from build123d import *

# Parameters (mm, degrees)
BOSS_EXTRU_1_DEPTH           = 10
BOSS_EXTRU_2_DEPTH           = 10
ESQUISSE4_R                  = 1.6
ENL_V_MAT_EXTRU_1_DEPTH      = 15
ESQUISSE5_R                  = 2.05
ENL_V_MAT_EXTRU_2_DEPTH      = 15
CONG_1_R                     = 2.5
ESQUISSE6_W                  = 10
ESQUISSE6_H                  = 2
BOSS_EXTRU_3_DEPTH           = 10
CHANFREIN1_SIZE              = 10
CONG_1_OF_SYM_TRIE1_R        = 2.5
CHANFREIN1_OF_SYM_TRIE1_SIZE = 10


with BuildPart() as part:
    # Esquisse2 → Boss.-Extru.1 (new body)
    with BuildSketch(Plane.XY):
        Polygon((125, 17.5), (125, 7.5), (20, 7.5), (20, 17.5), (15, 17.5), (15, 7.5), (0, 7.5), (0, -7.5), (125, -7.5), (125, -17.5), (130, -17.5), (130, 17.5), align=None)
    boss_extru_1 = extrude(amount=BOSS_EXTRU_1_DEPTH)

    # Esquisse3 → Boss.-Extru.2 (add)
    with BuildSketch(Plane.XY.offset(10)):
        Polygon((125, 7.5), (125, -7.5), (125, -17.5), (130, -17.5), (130, 17.5), (125, 17.5), align=None)
    boss_extru_2 = extrude(amount=BOSS_EXTRU_2_DEPTH)

    # Esquisse4 → Enlèv. mat.-Extru.1 (cut)
    with BuildSketch(Plane.ZY.offset(-15)):
        with Locations((5, 12.5)):
            Circle(ESQUISSE4_R)
    enl_v_mat_extru_1 = extrude(amount=-ENL_V_MAT_EXTRU_1_DEPTH, mode=Mode.SUBTRACT)

    # Esquisse5 → Enlèv. mat.-Extru.2 (cut)
    with BuildSketch(Plane.ZY.offset(-125)):
        with Locations(Location((10, 12.5, 0), (0, 0, 270))):
            Circle(ESQUISSE5_R)
        with Locations(Location((10, -12.5, 0), (0, 0, 180))):
            Circle(ESQUISSE5_R)
    enl_v_mat_extru_2 = extrude(amount=-ENL_V_MAT_EXTRU_2_DEPTH, mode=Mode.SUBTRACT)

    # Congé1
    cong_1_edges = [part.edges().sort_by_distance(p)[0] for p in [
        (127.5, 17.5, 0),
        (17.5, 17.5, 10),
        (127.5, -17.5, 0),
        (62.5, -7.5, 0),
        (7.5, 7.5, 0),
        (17.5, 17.5, 0),
        (72.5, 7.5, 0),
        (7.5, 7.5, 10),
        (62.5, -7.5, 10),
        (127.5, -17.5, 20),
        (127.5, 17.5, 20),
        (72.5, 7.5, 10),
    ]]
    fillet(cong_1_edges, radius=CONG_1_R)

    # Esquisse6 → Boss.-Extru.3 (add)
    with BuildSketch(Plane.ZY.offset(-125)):
        with Locations((15, 1)):
            Rectangle(ESQUISSE6_W, ESQUISSE6_H)
        with Locations((15, -1)):
            Rectangle(ESQUISSE6_W, ESQUISSE6_H)
    boss_extru_3 = extrude(amount=BOSS_EXTRU_3_DEPTH)

    # Chanfrein1
    chanfrein1_edges = [part.edges().sort_by_distance(p)[0] for p in [
        (115, 0, 20),
    ]]
    chamfer(chanfrein1_edges, length=CHANFREIN1_SIZE - 0.0001)  # a hair under: the kernel refuses the full size

    # Symétrie1: Boss.-Extru.1, Boss.-Extru.2, Enlèv. mat.-Extru.1, Enlèv. mat.-Extru.2, Boss.-Extru.3 across plane
    add(boss_extru_1.mirror(Plane(origin=(0, 0, 0), x_dir=(0, 0, 1), z_dir=(1, 0, 0))))
    add(boss_extru_2.mirror(Plane(origin=(0, 0, 0), x_dir=(0, 0, 1), z_dir=(1, 0, 0))))
    add(enl_v_mat_extru_1.mirror(Plane(origin=(0, 0, 0), x_dir=(0, 0, 1), z_dir=(1, 0, 0))), mode=Mode.SUBTRACT)
    add(enl_v_mat_extru_2.mirror(Plane(origin=(0, 0, 0), x_dir=(0, 0, 1), z_dir=(1, 0, 0))), mode=Mode.SUBTRACT)
    add(boss_extru_3.mirror(Plane(origin=(0, 0, 0), x_dir=(0, 0, 1), z_dir=(1, 0, 0))))

    # Congé1 of Symétrie1
    cong_1_of_sym_trie1_edges = [part.edges().sort_by_distance(p)[0] for p in [
        (-127.5, 17.5, 0),
        (-17.5, 17.5, 10),
        (-127.5, -17.5, 0),
        (-62.5, -7.5, 0),
        (-7.5, 7.5, 0),
        (-17.5, 17.5, 0),
        (-72.5, 7.5, 0),
        (-7.5, 7.5, 10),
        (-62.5, -7.5, 10),
        (-127.5, -17.5, 20),
        (-127.5, 17.5, 20),
        (-72.5, 7.5, 10),
    ]]
    fillet(cong_1_of_sym_trie1_edges, radius=CONG_1_OF_SYM_TRIE1_R)

    # Chanfrein1 of Symétrie1
    chanfrein1_of_sym_trie1_edges = [part.edges().sort_by_distance(p)[0] for p in [
        (-115, 0, 20),
    ]]
    chamfer(chanfrein1_of_sym_trie1_edges, length=CHANFREIN1_OF_SYM_TRIE1_SIZE - 0.0001)  # a hair under: the kernel refuses the full size


solid = part.part
The model under review builds one solid part; all positions refer to its coordinate system, in mm. A direction names the side the tool comes from. Give positions to 0.01 mm unless a question says otherwise; leave off trailing zeros. Order: outer loops, then holes, each group sorted by start corner. A loop starts at its lowest first (then second) coordinate and runs counter-clockwise, first axis right, second up. Notation, with made-up numbers: M -22,83 L -15,83 A17 cw -15,106 Z; hole C 63.5,-19 d1. An arc over 180 degrees is marked long. Answer in a Markdown table with one row per item. Add a question column.
1. For pin 1 Ø10 at (x, z) = (23.5, 10.5) entering from -Y; pin 2 Ø8 at (x, z) = (-121.5, 16) entering from +Y; pin 3 Ø12 at (x, z) = (62, 14) entering from +Y; pin 4 Ø5 at (x, z) = (-79, 6) entering from +Y, all flat-tipped, find the tip position at first contact; note any pin that passes through.
2. Machinability: for faces 1 (the flat face through (-121, 2, 14)), 2 (the flat face through (2, -7.5, 5)), 3 (the flat face through (73, 7.5, 5)), 4 (the cylindrical face through (-127.465, 14.127, 8.753)), which of the approach directions +Z, -Z, +X, -X, +Y, -Y give a long, thin tool a straight path to every point of the face, cutting with its end or side? Answer none if there is none.
3. Mouldability with a two-part tool opening along Y and no side actions: class faces 5 (the flat face through (-15, 11, 4)), 6 (the flat face through (121, -2, 14)), 7 (the cylindrical face through (127.465, 14.127, 8.753)) as released by +Y, released by -Y, zero draft, split by the parting line, or undercut.
4. Add section A-A on x = -54.5. State the section outline as (y, z) points, plus the area to 3 significant figures.
5. To check wall thickness, follow line 1 along Y through (x, z) = (-127.8, 10); line 2 along X through (y, z) = (15, 5.25); line 3 along X through (y, z) = (6, 12.25). State the ranges of each line that lie inside material, in increasing order.
The answers:
| question | item | result |
|---|---|---|
| 1 | pin 1 | y = -7.5 |
| 1 | pin 2 | y = 17.5 |
| 1 | pin 3 | y = 7.45 |
| 1 | pin 4 | y = 7.5 |
| 2 | face 1 | +Z, +Y |
| 2 | face 2 | +Z, -Z, -Y |
| 2 | face 3 | +Z, -Z, +Y |
| 2 | face 4 | -X |
| 3 | face 5 | zero draft |
| 3 | face 6 | released by -Y |
| 3 | face 7 | undercut |
| 4 | outline | M -7.5,2.5 A2.5 ccw -5,0 L 5,0 A2.5 ccw 7.5,2.5 L 7.5,7.5 A2.5 ccw 5,10 L -5,10 A2.5 ccw -7.5,7.5 Z |
| 4 | area | 145 mm2 |
| 5 | line 1 | -17.5 to -14.55, -10.45 to 10.45, 14.55 to 17.5 |
| 5 | line 2 | -130 to -125, -20 to -15, 15 to 20, 125 to 130 |
| 5 | line 3 | -130 to -125, 125 to 130 |
